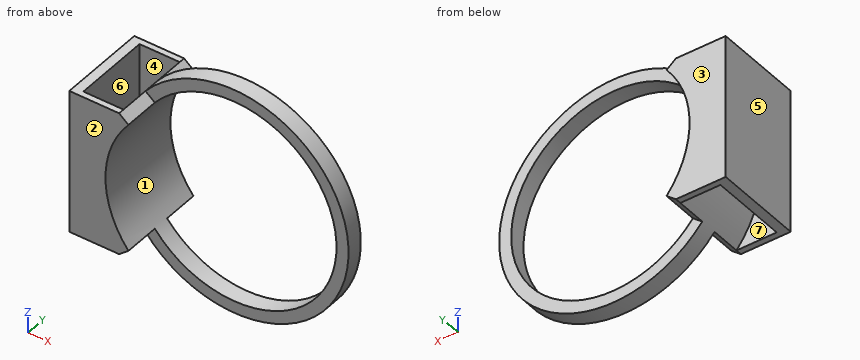
```python
from build123d import *

# Parameters (mm, degrees)
SKETCH_1_R          = 8.5
EXTRUDE_1_DEPTH     = 0.5
SKETCH_5_R          = 9.5
SKETCH_5_R_2        = 8.5
SKETCH_5_W          = 0.8
SKETCH_5_H          = 12
EXTRUDE_4_DEPTH     = 6.4
SKETCH_6_R          = 8.5
EXTRUDE_5_DEPTH     = 0.5
CUT_EXTRUDE_START   = -3
CUT_EXTRUDE_1_DEPTH = 3
CUT_EXTRUDE_2_DEPTH = 3


with BuildPart() as part:
    # 草图1 → 凸台-拉伸1 (new body)
    with BuildSketch(Plane(origin=(0, 0, 0), x_dir=(1, 0, 0), z_dir=(0, 1, 0))):
        with BuildLine():
            Line((-11.5, 6), (-11.5, -6))
            Line((-11.5, -6), (-7.365459931, -6))
            ThreePointArc((-7.365459931, -6), (9.5, 0), (-7.365459931, 6))
            Line((-7.365459931, 6), (-11.5, 6))
        make_face()
        with Locations(Location((0, 0, 0), (0, 0, 270))):
            Circle(SKETCH_1_R, mode=Mode.SUBTRACT)
    extrude(amount=EXTRUDE_1_DEPTH)

    # 草图5 → 凸台-拉伸4 (add)
    # profile 1 of 2: a face of its own
    with BuildSketch(Plane(origin=(0, 0.5, 0), x_dir=(1, 0, 0), z_dir=(0, 1, 0))):
        with Locations(Location((0, 0, 0), (0, 0, 140.833289284))):
            Circle(SKETCH_5_R)
        with Locations(Location((0, 0, 0), (0, 0, 270))):
            Circle(SKETCH_5_R_2, mode=Mode.SUBTRACT)
    # profile 2 of 2: a face of its own
    with BuildSketch(Plane(origin=(0, 0.5, 0), x_dir=(1, 0, 0), z_dir=(0, 1, 0))):
        with Locations((-11.1, 0)):
            Rectangle(SKETCH_5_W, SKETCH_5_H)
    extrude(amount=EXTRUDE_4_DEPTH)

    # 草图6 → 凸台-拉伸5 (add)
    with BuildSketch(Plane(origin=(0, 6.9, 0), x_dir=(1, 0, 0), z_dir=(0, 1, 0))):
        with BuildLine():
            Line((-11.5, 6), (-11.5, -6))
            Line((-11.5, -6), (-7.365459931, -6))
            ThreePointArc((-7.365459931, -6), (9.5, 0), (-7.365459931, 6))
            Line((-7.365459931, 6), (-11.5, 6))
        make_face()
        with Locations(Location((0, 0, 0), (0, 0, 270))):
            Circle(SKETCH_6_R, mode=Mode.SUBTRACT)
    extrude(amount=EXTRUDE_5_DEPTH)

    # 草图7 → 切除-拉伸1 (cut)
    with BuildSketch(Plane(origin=(0, 7.4, 0), x_dir=(1, 0, 0), z_dir=(0, 1, 0)).offset(CUT_EXTRUDE_START)):
        with BuildLine():
            Line((-7.365459931, 6), (-6.59014836, 5.368421053))
            ThreePointArc((-6.59014836, 5.368421053), (8.5, 0), (-6.59014836, -5.368421053))
            Line((-6.59014836, -5.368421053), (-7.365459931, -6))
            ThreePointArc((-7.365459931, -6), (9.5, 0), (-7.365459931, 6))
        make_face()
    extrude(amount=CUT_EXTRUDE_1_DEPTH, mode=Mode.SUBTRACT)

    # 草图8 → 切除-拉伸2 (cut)
    with BuildSketch(Plane(origin=(0, 0, 0), x_dir=(-1, 0, 0), z_dir=(0, -1, 0))):
        with BuildLine():
            Line((7.365459931, -6), (6.59014836, -5.368421053))
            ThreePointArc((6.59014836, -5.368421053), (-8.5, 0), (6.59014836, 5.368421053))
            Line((6.59014836, 5.368421053), (7.365459931, 6))
            ThreePointArc((7.365459931, 6), (-9.5, 0), (7.365459931, -6))
        make_face()
    extrude(amount=-CUT_EXTRUDE_2_DEPTH, mode=Mode.SUBTRACT)


solid = part.part
```
Can you work these out from the model? Positions are in its coordinate system, mm. Face numbers are marked on the shaded views. A direction names the side the tool comes from. Coordinates: 2 decimals unless noted, no trailing zeros. Write each loop counter-clockwise with the first axis right and the second up, starting at its lowest first coordinate (ties: lowest second). Pieces come first, ordered by that corner, then holes. Notation, with made-up numbers: M 52,62 L 96,62 A22 cw 96,83 Z; hole C -2,56.25 d4. An arc over 180 degrees is marked long. Write item = value, one per line. Start each with the question number.
Q1. If we section it at D-D, the plane y = 3.5: Write out the boundary of the cut face in (x, z), then the cut area to 3 significant figures.
Q2. If I drill on L1, parallel to X at y = 4, z = 1.5; L2, parallel to X at y = 3.5, z = -4; L3, parallel to X at y = 1.75, z = -4.5, over which ranges is the centre line in solid material (lowest first)? Write a range as [from, to].
Q3. If we section it at C-C, the plane y = 5.5: Write out the boundary of the cut face in (x, z).
Q4. If we section it at B-B, the plane z = 0: Write out the boundary of the cut face in (x, y), then the cut area to 3 significant figures.
Q5. If we section it at A-A, the plane x = 0: Write out the boundary of the cut face in (y, z).
Q6. Thinking about a two-plate mould opening in Y: for the marked faces 1, 2, 3 and 4, which applies, released by +Y, released by -Y, zero draft, split by the parting line, or undercut?
Q7. I'm going to push flat-ended pins straight in: pin 1 (1.5 mm diameter, centred on x = -8.5, y = 4.5, fed in from +Z); pin 2 (1.5 mm diameter, centred on x = -5.5, y = 3.5, fed in from +Z); pin 3 (1 mm diameter, centred on y = 4.5, z = 5.5, fed in from +X). Where does each tip first touch, or does it pass through?
Q8. On a 3-axis mill with a long thin cutter (end or side, diameter ignored), from which of +Z, -Z, +X, -X, +Y, -Y can I reach the whole of each face in a straight line? I mean the marked faces 5, 6 and 7. Say none if no direction works.
Check sheet entries:
q1.outline = M -11.5,-6 L -10.7,-6 L -10.7,6 L -11.5,6 Z; C 0,0 d19; hole C 0,0 d17
q1.area = 66.1 mm²
q2.L1 = [-11.5, -10.7], [-9.38, -8.37], [8.37, 9.38]
q2.L2 = [-11.5, -10.7], [-8.62, -7.5], [7.5, 8.62]
q2.L3 = [-11.5, -10.7], [-8.37, -7.21]
q3.outline = M -11.5,-6 L -10.7,-6 L -10.7,6 L -11.5,6 Z; M -7.37,-6 L -6.59,-5.37 A8.5 cw -6.59,5.37 L -7.37,6 A9.5 ccw Z
q4.outline = M -11.5,0 L -8.5,0 L -8.5,7.4 L -11.5,7.4 Z; M 8.5,3 L 9.5,3 L 9.5,4.4 L 8.5,4.4 Z; hole M -10.7,0.5 L -9.5,0.5 L -9.5,6.9 L -10.7,6.9 Z
q4.area = 15.9 mm²
q5.outline = M 3,-9.5 L 4.4,-9.5 L 4.4,-8.5 L 3,-8.5 Z; M 3,8.5 L 4.4,8.5 L 4.4,9.5 L 3,9.5 Z
q6.face_1 = zero draft
q6.face_2 = released by -Y
q6.face_3 = released by +Y
q6.face_4 = undercut
q7.pin_1 = 5.49
q7.pin_2 = 8.23
q7.pin_3 = 8.07
q8.face_5 = +Z, -Z, -X, +Y, -Y
q8.face_6 = +Z, -Z
q8.face_7 = none
